Autodesk Inventor part; units mm, degrees
ref_plane "YZ Plane" through (0, 0, 0) normal (1, 0, 0) x (0, 1, 0)
ref_plane "XZ Plane" through (0, 0, 0) normal (0, 1, 0) x (-1, 0, 0)
ref_plane "XY Plane" through (0, 0, 0) normal (0, 0, 1) x (1, 0, 0)
sketch "Skizze1" plane through (0, 0, 0) normal (0, 0, 1) x (1, 0, 0)
  circle A0 centre (0, 0) radius 2.5
  dimension "d0" = 5
extrude "Extrusion1" add sketch "Skizze1" along normal mid plane 469
sketch "Skizze2" plane through (0, 0, 234.5) normal (0, 0, 1) x (1, 0, 0)
  line L0 (-2.3094, 4) -> (2.3094, 4)
  line L1 (2.3094, 4) -> (4.6188, 0)
  line L2 (4.6188, 0) -> (2.3094, -4)
  line L3 (2.3094, -4) -> (-2.3094, -4)
  line L4 (-2.3094, -4) -> (-4.6188, 0)
  line L5 (-4.6188, 0) -> (-2.3094, 4)
  point P0 (0, 0)
  point P1 (0, 0)
  dimension "d3" = 8
extrude "Extrusion2" add sketch "Skizze2" against normal blind 20
mirror "Spiegeln1" about plane through (0, 0, 0) normal (0, 0, 1) of "Extrusion2"
properties part number "Door Axis" material "Edelstahl"
Input: part model. Units: mm. Frame: model coordinates. Coordinates: 2 decimals unless noted, no trailing zeros. Loops run counter-clockwise (first coordinate to the right, second up) from the corner with the lowest first, then second, coordinate; pieces in that order, holes last. Notation, with made-up numbers: M 53.25,13 L 65.25,13 A24 ccw 65.25,37 Z; hole C -32,77.5 d11. An arc over 180 degrees is marked long. Answer in a Markdown table with one row per item.
1. Section A-A, the plane x = 0. Output: boundary loops of the cut face in (y, z).
Response:
| item | result |
|---|---|
| outline | M -4,-234.5 L 4,-234.5 L 4,-214.5 L 2.5,-214.5 L 2.5,214.5 L 4,214.5 L 4,234.5 L -4,234.5 L -4,214.5 L -2.5,214.5 L -2.5,-214.5 L -4,-214.5 Z |
2. Material intervals for line 1 (Z direction, x = 1.5, y = -3); line 2 (Y direction, x = -0.5, z = 20); line 3 (X direction, y = -0.25, z = -27), sorted ascending.
Response:
| item | result |
|---|---|
| line 1 | z = -234.5 to -214.5, 214.5 to 234.5 |
| line 2 | y = -2.45 to 2.45 |
| line 3 | x = -2.49 to 2.49 |
3. First-contact query: pin 1 (4 mm diameter, centred on y = 0.5, z = 6.5, fed in from +X); pin 2 (2 mm diameter, centred on x = 1, z = 62, fed in from -Y); pin 3 (1 mm diameter, centred on y = -1.5, z = -115.5, fed in from +X). Flat tips, straight axial feed; report the tip coordinate or a pass-through.
Response:
| item | result |
|---|---|
| pin 1 | stops at x = 2.5 |
| pin 2 | stops at y = -2.5 |
| pin 3 | stops at x = 2.29 |
4. Draft query along Z for faces 1 (the flat face through (0, 0, 234.5)), 2 (the flat face through (2, 2, 214.5)), 3 (the flat face through (0, 0, -234.5)). Return one class per face: pulls with the +Z half, pulls with the -Z half, needs draft (parallel to the pull), parting line crosses it, or undercut.
Response:
| item | result |
|---|---|
| face 1 | pulls with the +Z half |
| face 2 | undercut |
| face 3 | pulls with the -Z half |
5. Section B-B, the plane z = 147. Output: boundary loops of the cut face in (x, y), then the cut area to 3 significant figures.
Response:
| item | result |
|---|---|
| outline | C 0,0 d5 |
| area | 19.6 mm2 |
